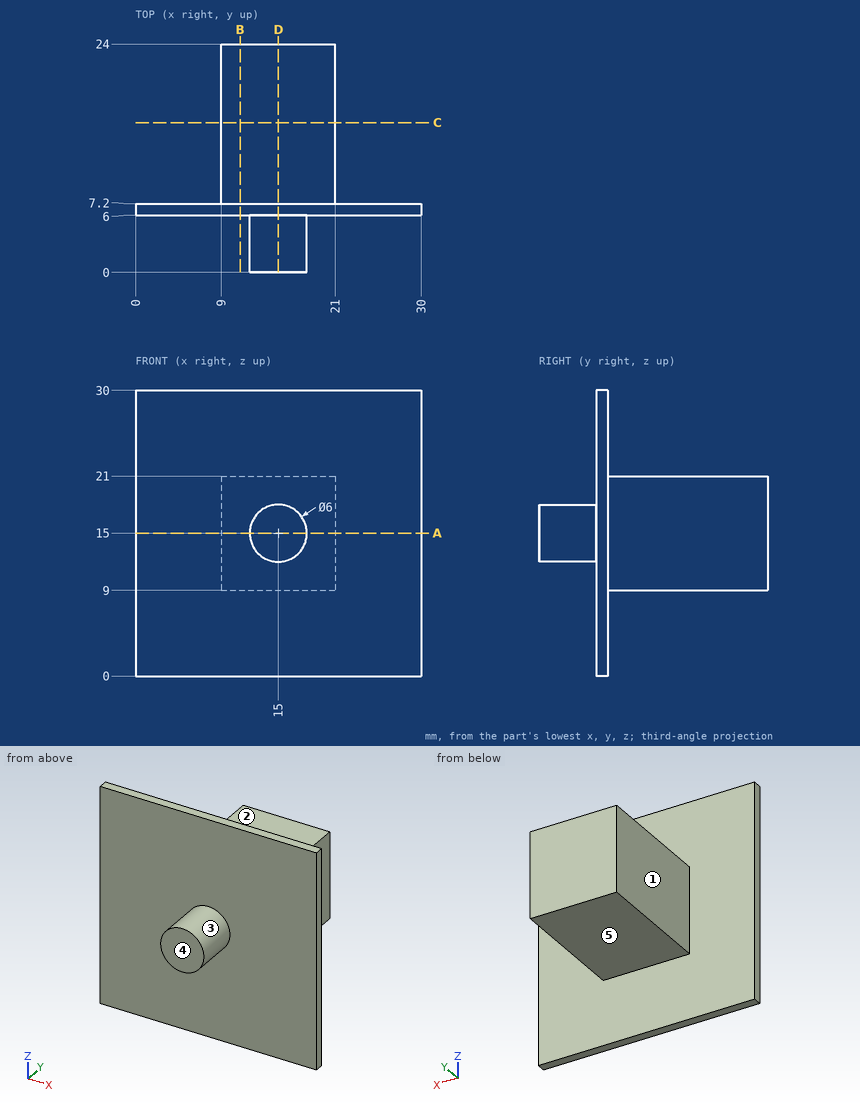
Here's the drawing with two shaded views (mm, measured from the low corner). I have some questions. A direction names the side the tool comes from. Give positions to 0.01 mm unless a question says otherwise; leave off trailing zeros. Loops run counter-clockwise (first coordinate to the right, second up) from the corner with the lowest first, then second, coordinate; pieces in that order, holes last. Notation, with made-up numbers: (-39.75, 67) -> (4.25, 67) arc R19 cw to (4.25, 94) -> close; hole circle Ø7 at (-35, 75). An arc over 180 degrees is marked (long way). Answer as a JSON object with one key per item and string values. Group by question number.
Item 1: Will these pins go through, and if not, where does the flat tip stop? pin 1 (12 mm diameter, centred on x = 7.5, z = 4, fed in from -Y); pin 2 (3.5 mm diameter, centred on y = 14.5, z = 17, fed in from -X); pin 3 (13 mm diameter, centred on x = 15.5, y = 14, fed in from +Z).
Item 2: Imagine slicing it at A-A on z = 15. Write out the boundary of the cut face in (x, y).
Item 3: Imagine slicing it at D-D on x = 15. Write out the boundary of the cut face in (y, z).
Item 4: Imagine slicing it at B-B on x = 11. Write out the boundary of the cut face in (y, z).
Item 5: I need wall thicknesses on L1, parallel to Y at x = 6.5, z = 27.75; L2, parallel to X at y = 17.75, z = 20.5; L3, parallel to Y at x = 9.25, z = 14.25. Which ranges of each line are inside material? Lowest first, please.
Item 6: Imagine slicing it at C-C on y = 15.75. Write out the boundary of the cut face in (x, z), then the cut area to 3 significant figures.
Item 7: On a 3-axis mill with a long thin cutter (end or side, diameter ignored), from which of +Z, -Z, +X, -X, +Y, -Y can I reach the whole of each face in a straight line? I mean the marked faces 1, 2, 3, 4 and 5. Say none if no direction works.
Answer list:
{
 "1": {"pin 1": "stops at y = 6", "pin 2": "stops at x = 9", "pin 3": "stops at z = 21"},
 "2": {"outline": "(0, 6) -> (12, 6) -> (12, 0) -> (18, 0) -> (18, 6) -> (30, 6) -> (30, 7.2) -> (21, 7.2) -> (21, 24) -> (9, 24) -> (9, 7.2) -> (0, 7.2) -> close"},
 "3": {"outline": "(0, 12) -> (6, 12) -> (6, 0) -> (7.2, 0) -> (7.2, 9) -> (24, 9) -> (24, 21) -> (7.2, 21) -> (7.2, 30) -> (6, 30) -> (6, 18) -> (0, 18) -> close"},
 "4": {"outline": "(6, 0) -> (7.2, 0) -> (7.2, 9) -> (24, 9) -> (24, 21) -> (7.2, 21) -> (7.2, 30) -> (6, 30) -> close"},
 "5": {"L1": "y = 6 to 7.2", "L2": "x = 9 to 21", "L3": "y = 6 to 24"},
 "6": {"outline": "(9, 9) -> (21, 9) -> (21, 21) -> (9, 21) -> close", "area": "144 mm2"},
 "7": {"face 1": "+Z, -Z, -X, +Y", "face 2": "+Z, +X, -X, +Y", "face 3": "-Y", "face 4": "+Z, -Z, +X, -X, -Y", "face 5": "-Z, +X, -X, +Y"}
}
